```python
from build123d import *

# Parameters (mm, degrees)
F0_R     = 110
F0_R_2   = 1.6
F1_DEPTH = 3
F2_SIZE  = 2.6


with BuildPart() as f1:
    # F0 (on Top) → F1 (new body)
    with BuildSketch(Plane.XY):
        Circle(F0_R)
        with Locations((-91.105872, -52.6)):
            Circle(F0_R_2, mode=Mode.SUBTRACT)
        with Locations((0, -105.2)):
            Circle(F0_R_2, mode=Mode.SUBTRACT)
        with Locations((91.105872, -52.6)):
            Circle(F0_R_2, mode=Mode.SUBTRACT)
        with Locations((-91.105872, 52.6)):
            Circle(F0_R_2, mode=Mode.SUBTRACT)
        with Locations((91.105872, 52.6)):
            Circle(F0_R_2, mode=Mode.SUBTRACT)
        with Locations((0, 105.2)):
            Circle(F0_R_2, mode=Mode.SUBTRACT)
    extrude(amount=F1_DEPTH)

    # F2
    f2_edges = [f1.edges().sort_by_distance(p)[0] for p in [
        (-92.705872, 52.6, 3),
        (-1.6, 105.2, 3),
        (89.505872, 52.6, 3),
        (89.505872, -52.6, 3),
        (-1.6, -105.2, 3),
        (-92.705872, -52.6, 3),
    ]]
    chamfer(f2_edges, length=F2_SIZE)


solid = f1.part
```
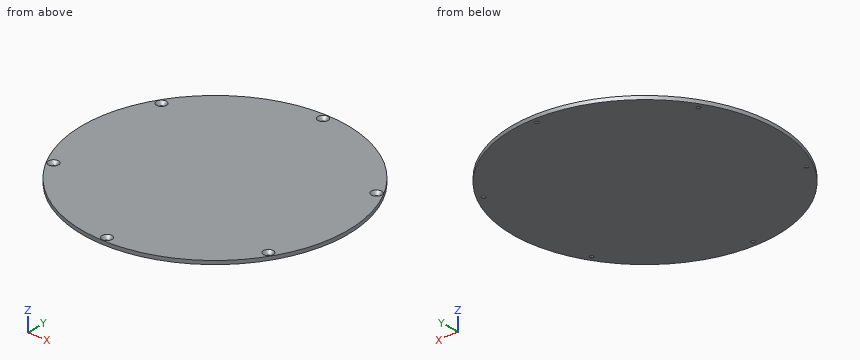
Model file for the job. Use its own axes, mm. Coordinates: 2 decimals unless noted, no trailing zeros. Order: outer loops, then holes, each group sorted by start corner. A loop starts at its lowest first (then second) coordinate and runs counter-clockwise, first axis right, second up. Notation, with made-up numbers: (1.5, 8) -> (51.5, 8) arc R21 cw to (51.5, 13) -> close; hole circle Ø7 at (-7, -15.75). An arc over 180 degrees is marked (long way). Return JSON: item names as keys, results as strings.
Item 1: Wall check: line 1 along Y through (x, z) = (0, 0.2); line 2 along Y through (x, z) = (26.5, 2.5); line 3 along Y through (x, z) = (83, 2.45). Give the ranges that are in metal, low to high. Write a range as from..to.
Model answer:
{"line 1": "y = -110..-106.8, -103.6..103.6, 106.8..110", "line 2": "y = -106.76..106.76", "line 3": "y = -72.19..72.19"}
Item 2: Slice it at C-C (x = 34). Write the cut outline in (y, z).
Model answer:
{"outline": "(-104.61, 0) -> (104.61, 0) -> (104.61, 3) -> (-104.61, 3) -> close"}
Item 3: Slice it at A-A (z = 1.85). Write the cut outline in (x, y).
Model answer:
{"outline": "circle Ø220 at (0, 0); hole circle Ø6.1 at (-91.11, -52.6); hole circle Ø6.1 at (-91.11, 52.6); hole circle Ø6.1 at (0, -105.2); hole circle Ø6.1 at (0, 105.2); hole circle Ø6.1 at (91.11, -52.6); hole circle Ø6.1 at (91.11, 52.6)"}
Item 4: Slice it at B-B (y = -35). Write the cut outline in (x, z), then the cut area to 3 significant figures.
Model answer:
{"outline": "(-104.28, 0) -> (104.28, 0) -> (104.28, 3) -> (-104.28, 3) -> close", "area": "626 mm²"}
Item 5: Pin check, flat tips, straight feed: P1, Ø5, axis at x = -91.11, y = 52.6, coming from the +Z side; P2, Ø4, axis at x = 0, y = -105.2, coming from the +Z side. Stop position of each tip, or through.
Model answer:
{"P1": "stops at z = 1.3", "P2": "stops at z = 0.8"}
